Autodesk Inventor part; units mm, degrees
ref_plane "YZ Plane" through (0, 0, 0) normal (1, 0, 0) x (0, 1, 0)
ref_plane "XZ Plane" through (0, 0, 0) normal (0, 1, 0) x (-1, 0, 0)
ref_plane "XY Plane" through (0, 0, 0) normal (0, 0, 1) x (1, 0, 0)
sketch "Sketch1" plane through (0, 0, 0) normal (0, 1, 0) x (-1, 0, 0)
  line L0 (-3.3361, 9.3016) -> (3.4264, 9.3016)
  line L1 (3.4264, 9.3016) -> (3.4264, -8.4784)
  line L2 (3.4264, -8.4784) -> (-3.3361, -8.4784)
  line L3 (-3.3361, -8.4784) -> (-3.3361, 9.3016)
  line L4 (2.4264, -7.4784) -> (2.4264, 8.3016)
  line L5 (2.4264, 8.3016) -> (-2.3361, 8.3016)
  line L6 (-2.3361, 8.3016) -> (-2.3361, -7.4784)
  line L7 (-2.3361, -7.4784) -> (2.4264, -7.4784)
  point P0 (0, 0)
  dimension "d0" = 17.78
  dimension "d1" = 6.7625
  dimension "d2" = 1
extrude "Extrusion1" add sketch "Sketch1" along normal blind 4
fillet "Fillet1" radius 1 8 edges at (-3.4264, 2, 9.3016) (-3.4264, 2, -8.4784) (3.3361, 2, -8.4784) (3.3361, 2, 9.3016) (2.3361, 2, 8.3016) (-2.4264, 2, 8.3016) (-2.4264, 2, -7.4784) (2.3361, 2, -7.4784)
sketch "Sketch2" plane through (-2.4264, 0, -5.9384) normal (-1, 0, 0) x (0, 0, 1)
  circle A0 centre (0, 2) radius 2.54
  circle A1 centre (12.7, 2) radius 2.54
  line L0 (-1.54, 4) -> (14.24, 4)
  line L1 (15.24, 0) -> (15.24, 4)
  line L2 (15.24, 2) -> (-2.54, 2) construction
  line L3 (-2.54, 0) -> (-2.54, 4)
  dimension "d6" = 5.08
  dimension "d7" = 12.7
surface extrude "ExtrusionSrf1" sketch "Sketch2" along normal up to surface (1 mm away) shown yes curves A0
surface extrude "ExtrusionSrf2" sketch "Sketch2" along normal up to surface (1 mm away) shown yes curves A1
properties part number "ziptie" material "Acetal Resin, Black"
Work out the finished part from the listing and answer in its coordinate system (mm). A direction names the side the tool comes from. Round coordinates to 2 decimals unless told otherwise and drop trailing zeros. Write each loop counter-clockwise with the first axis right and the second up, starting at its lowest first coordinate (ties: lowest second). Pieces come first, ordered by that corner, then holes. Notation, with made-up numbers: (38.5, 64) -> (88.5, 64) arc R16 cw to (88.5, 73) -> close; hole circle Ø4 at (63.25, -9.75). An arc over 180 degrees is marked (long way). Write each question's results on one line, items separated by ' | '.
Q1. Section A-A, the plane x = -0.5 is taken. Write down the section's boundary in (y, z).
Data:
outline: (0, -8.48) -> (4, -8.48) -> (4, -7.48) -> (0, -7.48) -> close; (0, 8.3) -> (4, 8.3) -> (4, 9.3) -> (0, 9.3) -> close
Q2. Section D-D, the plane x = 3 is taken. Write down the section's boundary in (y, z).
Data:
outline: (0, -8.23) -> (4, -8.23) -> (4, 9.05) -> (0, 9.05) -> close
Q3. Which of the six approach directions +Z, -Z, +X, -X, +Y, -Y give full straight-line access (tool end or side, diameter ignored) to faces 1 (the flat face through (-3.426, 2, 1)), 2 (the flat face through (0, 2, 8.302))?
Data:
face 1: +Z, -Z, -X, +Y, -Y | face 2: +Y, -Y
Q4. Straight lines are drawn through the part: line 1 along X through (y, z) = (1.9, -1.5); line 2 along Z through (x, y) = (0.5, 1.75); line 3 along X through (y, z) = (3.5, -7.25). For each, find the intervals that lie inside material, in ascending order. Write a range as [from, to].
Data:
line 1: [-3.43, -2.43], [2.34, 3.34] | line 2: [-8.48, -7.48], [8.3, 9.3] | line 3: [-3.43, -2.06], [1.97, 3.34]
Q5. Determine the mould class of faces 3 (the flat face through (-3, 0, 2)), 4 (the cylindrical face through (-3.14, 2.03, 9)), 5 (the cylindrical face through (-2.14, 2.03, 8)) for opening direction X: released by +X, released by -X, zero draft, split by the parting line, or undercut.
Data:
face 3: zero draft | face 4: released by -X | face 5: undercut
Q6. Section C-C, the plane z = -2.25 is taken. Write down the section's boundary in (x, y), then the cut area to 3 significant figures.
Data:
outline: (-3.43, 0) -> (-2.43, 0) -> (-2.43, 4) -> (-3.43, 4) -> close; (2.34, 0) -> (3.34, 0) -> (3.34, 4) -> (2.34, 4) -> close | area: 8.00 mm^2
Q7. Section B-B, the plane y = 1.2 is taken. Write down the section's boundary in (x, z), then the cut area to 3 significant figures.
Data:
outline: (-3.43, -7.48) arc R1 ccw to (-2.43, -8.48) -> (2.34, -8.48) arc R1 ccw to (3.34, -7.48) -> (3.34, 8.3) arc R1 ccw to (2.34, 9.3) -> (-2.43, 9.3) arc R1 ccw to (-3.43, 8.3) -> close; hole (-2.43, -6.48) arc R1 ccw to (-1.43, -7.48) -> (1.34, -7.48) arc R1 ccw to (2.34, -6.48) -> (2.34, 7.3) arc R1 ccw to (1.34, 8.3) -> (-1.43, 8.3) arc R1 ccw to (-2.43, 7.3) -> close | area: 45.1 mm^2
